Verification items for the finished model (mm, model axes). Round coordinates to 2 decimals unless told otherwise and drop trailing zeros. Write each loop counter-clockwise with the first axis right and the second up, starting at its lowest first coordinate (ties: lowest second). Pieces come first, ordered by that corner, then holes. Notation, with made-up numbers: M 44,-39.75 L 84,-39.75 A17 cw 84,-9.75 Z; hole C 4.25,-16.75 d1. An arc over 180 degrees is marked long. Write each question's results on one line, items separated by ' | '.
Autodesk Inventor part; units mm, degrees
ref_plane "YZ Plane" through (0, 0, 0) normal (1, 0, 0) x (0, 1, 0)
ref_plane "XZ Plane" through (0, 0, 0) normal (0, 1, 0) x (-1, 0, 0)
ref_plane "XY Plane" through (0, 0, 0) normal (0, 0, 1) x (1, 0, 0)
sketch "Sketch1" plane through (0, 0, 0) normal (0, 1, 0) x (-1, 0, 0)
  line L0 (0, 0) -> (0, -3)
  line L1 (-250, -38) -> (-250, -78)
  line L2 (0, 0) -> (-20, 0)
  line L3 (-50, 0) -> (-50, -3)
  line L4 (-50, 0) -> (-70, 0)
  line L5 (-70, 0) -> (-70, -3)
  line L6 (-100, 0) -> (-100, -3)
  line L7 (-100, 0) -> (-120, 0)
  line L8 (-120, 0) -> (-120, -3)
  line L9 (-150, 0) -> (-150, -3)
  line L10 (-150, 0) -> (-170, 0)
  line L11 (-170, 0) -> (-170, -3)
  line L12 (-200, 0) -> (-200, -3)
  line L13 (-200, 0) -> (-220, 0)
  line L14 (-220, 0) -> (-220, -3)
  line L15 (-20, 0) -> (-20, -3)
  line L16 (-250, -58) -> (-250, -78)
  line L17 (-250, -78) -> (-247, -78)
  line L18 (-247, -78) -> (-247, -113)
  line L19 (-250, -58) -> (-250, -38)
  line L20 (-250, -38) -> (-247, -38)
  line L21 (-247, -38) -> (-247, -3)
  line L22 (-220, -3) -> (-247, -3)
  line L23 (-170, -3) -> (-200, -3)
  line L24 (-120, -3) -> (-150, -3)
  line L25 (-20, -3) -> (-50, -3)
  line L26 (-70, -3) -> (-100, -3)
  line L27 (0, -116) -> (0, -113)
  line L28 (0, -116) -> (-20, -116)
  line L29 (-50, -116) -> (-50, -113)
  line L30 (-50, -116) -> (-70, -116)
  line L31 (-70, -116) -> (-70, -113)
  line L32 (-100, -116) -> (-100, -113)
  line L33 (-100, -116) -> (-120, -116)
  line L34 (-120, -116) -> (-120, -113)
  line L35 (-150, -116) -> (-150, -113)
  line L36 (-150, -116) -> (-170, -116)
  line L37 (-170, -116) -> (-170, -113)
  line L38 (-200, -116) -> (-200, -113)
  line L39 (-200, -116) -> (-220, -116)
  line L40 (-220, -116) -> (-220, -113)
  line L41 (-20, -116) -> (-20, -113)
  line L42 (-3, -58) -> (-3, -78)
  line L43 (-3, -78) -> (0, -78)
  line L44 (-3, -58) -> (-3, -38)
  line L45 (-3, -38) -> (0, -38)
  line L46 (0, -113) -> (0, -78)
  line L47 (0, -38) -> (0, -3)
  line L48 (-50, -113) -> (-20, -113)
  line L49 (-100, -113) -> (-70, -113)
  line L50 (-150, -113) -> (-120, -113)
  line L51 (-247, -113) -> (-220, -113)
  line L52 (-200, -113) -> (-170, -113)
  line L53 (-230, -60) -> (-205, -60)
  line L54 (-205, -60) -> (-205, -63)
  line L55 (-205, -63) -> (-230, -63)
  line L56 (-230, -63) -> (-230, -60)
  line L57 (-162, -60) -> (-137, -60)
  line L58 (-137, -60) -> (-137, -63)
  line L59 (-137, -63) -> (-162, -63)
  line L60 (-162, -63) -> (-162, -60)
  dimension "d2" = 110
  dimension "d3" = 20
  dimension "d4" = 20
  dimension "d5" = 20
  dimension "d7" = 20
  dimension "d8" = 20
  dimension "d9" = 20
  dimension "d10" = 3
  dimension "d11" = 20
  dimension "d12" = 3
  dimension "d13" = 250
  dimension "d14" = 30
  dimension "d15" = 30
  dimension "d16" = 30
  dimension "d17" = 30
  dimension "d23" = 25
  dimension "d24" = 3
  dimension "d25" = 43
  dimension "d26" = 25
  dimension "d27" = 3
  dimension "d28" = 57
  dimension "d31" = 17
  dimension "d32" = 2
  dimension "d33" = 3
  dimension "d34" = 40
  dimension "d35" = 110
extrude "Extrusion2" add sketch "Sketch1" along normal blind 3
properties part number "latOpSupp"
1) Sectioned sample at A-A, the plane x = 142. Record the cut outline in (y, z).
Calculated:
outline: M 0,-113 L 3,-113 L 3,-63 L 0,-63 Z; M 0,-60 L 3,-60 L 3,-3 L 0,-3 Z
2) Sectioned sample at C-C, the plane x = 90.5. Record the cut outline in (y, z).
Calculated:
outline: M 0,-113 L 3,-113 L 3,-3 L 0,-3 Z
3) Sectioned sample at B-B, the plane y = 2.1. Count the separate pieces of the cut face and the enclosed holes in it, and give its area (3 significant figures).
Calculated:
separate pieces: 1 | enclosed holes: 2 | area: 27,600 mm²
4) Material ranges on line 1 (Z direction, x = 140, y = 2.2); line 2 (Z direction, x = 209, y = 1.85); line 3 (X direction, y = 2.3, z = -5), recorded low to high. Write a range as [from, to].
Calculated:
line 1: z = [-113, -63], [-60, -3] | line 2: z = [-116, -63], [-60, 0] | line 3: x = [0, 247]
5) Depth check by flat-ended pin: P1, Ø1.5, axis at x = 139.5, y = 1.5, coming from the -Z side; P2, Ø1.5, axis at y = 1, z = -1, coming from the +X side; P3, Ø0.9, axis at x = 36.5, y = 2, coming from the +Z side. Enter the tip coordinate at first touch or a pass-through.
Calculated:
P1: stops at z = -113 | P2: stops at x = 220 | P3: stops at z = -3
